from build123d import *

# Parameters (mm, degrees)
F0_W     = 13.4654790163
F0_H     = 6.7327402066
F0_H_2   = 6.5761648584
F0_W_2   = 22.2336961131
F0_H_3   = 13.3089050651
F0_W_3   = 24.73890463
F0_H_4   = 0.1565753482
F1_DEPTH = 25.4


with BuildPart() as f1:
    # F0 (on Front) → F1 (new body)
    with BuildSketch(Plane.XZ):
        Polygon((-38.204383105, 6.5761648584), (-38.204383105, 13.3089050651), (-24.7389040887, 13.3089050651), (-24.7389040887, 15.8141106367), (-38.8306863606, 15.8141106367), (-38.8306863606, 6.5761648584), align=None)
        with Locations((-31.4716435969, 9.9425349617)):
            Rectangle(F0_W, F0_H)
        Polygon((5.413e-07, 13.3089050651), (-24.7389040887, 13.3089050651), (-24.7389040887, 6.5761648584), (-24.7389040887, 0), (5.413e-07, 0), align=None)
        with Locations((-31.4716435969, 3.2880824292)):
            Rectangle(F0_W, F0_H_2)
        with Locations((11.1168485979, 6.6544525325)):
            Rectangle(F0_W_2, F0_H_3)
        Polygon((-38.8306863606, 15.8141106367), (-24.7389040887, 15.8141106367), (-11.899725534, 15.8141106367), (-11.899725534, 52.1395914257), (-38.8306863606, 52.1395914257), align=None)
        with Locations((-12.3694517737, -0.0782876741)):
            Rectangle(F0_W_3, F0_H_4)
    extrude(amount=F1_DEPTH)


solid = f1.part
Check sheet for the modelled part. Datum: model origin and axes. Units: mm. A direction names the side the tool comes from. Give positions to 0.01 mm unless a question says otherwise; leave off trailing zeros. Order: outer loops, then holes, each group sorted by start corner. A loop starts at its lowest first (then second) coordinate and runs counter-clockwise, first axis right, second up. Notation, with made-up numbers: (-13, -19) - (4, -19) arc R17 cw to (4, -14) - close; hole circle Ø5 at (27.5, 69.5). An arc over 180 degrees is marked (long way). Answer as CSV lines item,"result".
1. Scan lines: probe 1 along Z at (x, y) = (-24, -15); probe 2 along X at (y, z) = (-14.5, 16); probe 3 along Z at (x, y) = (-31, -15.5). Record each from-to range of solid material in increasing order. Write a range as from..to.
Result sheet:
probe 1,"-0.16..13.31, 15.81..52.14"
probe 2,"-38.83..-11.9"
probe 3,"0..52.14"
2. Go/stop test with flat-tipped pins: P1, Ø7.5, axis at x = 7, y = -17, coming from the +Z side; P2, Ø1.5, axis at x = -27, y = -7, coming from the -Z side; P3, Ø1.3, axis at y = -12.5, z = 15, coming from the +X side; P4, Ø8, axis at x = -6.5, z = 28, coming from the -Y side (1 decimal). Record where each tip stops, or that it passes through.
Result sheet:
P1,"z = 13.31"
P2,"z = 0"
P3,"x = -24.74"
P4,"through"
3. Section check D-D (z = 15). Record the boundary of the cut face in (x, y), then the cut area to 3 significant figures.
Result sheet:
outline,"(-38.83, -25.4) - (-24.74, -25.4) - (-24.74, 0) - (-38.83, 0) - close"
area,"358 mm²"
4. Section check A-A (x = -15). Record the boundary of the cut face in (y, z).
Result sheet:
outline,"(-25.4, -0.16) - (0, -0.16) - (0, 13.31) - (-25.4, 13.31) - close; (-25.4, 15.81) - (0, 15.81) - (0, 52.14) - (-25.4, 52.14) - close"
5. Section check B-B (y = -19). Record the boundary of the cut face in (x, z).
Result sheet:
outline,"(-38.83, 6.58) - (-38.2, 6.58) - (-38.2, 0) - (-24.74, 0) - (-24.74, -0.16) - (0, -0.16) - (0, 0) - (22.23, 0) - (22.23, 13.31) - (-24.74, 13.31) - (-24.74, 15.81) - (-11.9, 15.81) - (-11.9, 52.14) - (-38.83, 52.14) - close"
6. Tool access check on faces 1 (the face through (-32, -13, 0)), 2 (the face through (11, -13, 0)), 3 (the face through (-38.831, -13, 30)), 4 (the face through (-11.9, -13, 34)), 5 (the face through (-2, -13, 13.309)). Record the directions out of +Z, -Z, +X, -X, +Y, -Y that give a thin tool (end or side, any length) a straight path to the whole face; none if there is none.
Result sheet:
face 1,"-Z, -X, +Y, -Y"
face 2,"-Z, +X, +Y, -Y"
face 3,"+Z, -Z, -X, +Y, -Y"
face 4,"+Z, +X, +Y, -Y"
face 5,"+X, +Y, -Y"
7. Section check C-C (z = 25). Record the boundary of the cut face in (x, y), then the cut area to 3 significant figures.
Result sheet:
outline,"(-38.83, -25.4) - (-11.9, -25.4) - (-11.9, 0) - (-38.83, 0) - close"
area,"684 mm²"
